from build123d import *

# Parameters (mm, degrees)
F4_D     = 2.5
F4_DEPTH = 8
F4_START = 17.6049004
F4_TIP   = 0.7510757738


with BuildPart() as f1:
    # F0 (on Front) → F1 (revolve)
    with BuildSketch(Plane.XZ):
        Polygon((-7.5, 3), (13.5, 3), (13.5, 4), (7.5, 4), (7.5, 10), (5.75, 10), (5.75, 7.5), (-5.75, 7.5), (-5.75, 10), (-7.5, 10), align=None)
    revolve(axis=Axis((1.1428869498, 0, 0), (1, 0, 0)))

    # F4
    # its depths count from where the whole tool has entered the part; down to there all is cleared
    with Locations(Plane.XY.offset(25)):
        with Locations((0, 0)):
            Hole(F4_D / 2, depth=F4_START)
    with Locations(Plane.XY.offset(25).offset(-F4_START)):
        with Locations((0, 0)):
            Hole(F4_D / 2, depth=F4_DEPTH)
            with Locations((0, 0, -(F4_DEPTH + F4_TIP / 2))):  # 118° drill point
                Cone(0, F4_D / 2, F4_TIP, mode=Mode.SUBTRACT)


solid = f1.part
Work out the finished part from the listing and answer in its coordinate system (mm). A direction names the side the tool comes from. Give positions to 0.01 mm unless a question says otherwise; leave off trailing zeros. Order: outer loops, then holes, each group sorted by start corner. A loop starts at its lowest first (then second) coordinate and runs counter-clockwise, first axis right, second up. Notation, with made-up numbers: M -38.5,78.5 L -4.5,78.5 A30 cw -4.5,112.5 Z; hole C 56.25,27 d8. An arc over 180 degrees is marked long. Return JSON: item names as keys, results as strings.
Q1. The mould has two halves that part along Z. Classify faces 6 (the face through (6.61, 9.76, -2.17)), 7 (the face through (7.5, -0.1, -4.3)), 8 (the face through (3.1, 1.8, -2.4)): pulls with the +Z half, pulls with the -Z half, needs draft (parallel to the pull), parting line crosses it, or undercut.
Answer below:
{"face 6": "parting line crosses it", "face 7": "needs draft", "face 8": "undercut"}
Q2. Which of the six approach directions +Z, -Z, +X, -X, +Y, -Y give full straight-line access (tool end or side, diameter ignored) to faces 1 (the face through (-6.64, 9.76, -2.17)), 2 (the face through (10.458, 3.905, -0.867)), 3 (the face through (-0.59, 1.1, 5.08)), 4 (the face through (-5.75, -7, -4)), 5 (the face through (-7.5, -2.4, 2.1))?
Answer below:
{"face 1": "+X, -X", "face 2": "+X", "face 3": "+Z", "face 4": "none", "face 5": "+Z, -Z, -X, +Y, -Y"}
Q3. Each of these flat-tipped pins is pushed along its axis until it touches: pin 1 (6 mm diameter, centred on x = 1, z = -3.5, fed in from -Y); pin 2 (4 mm diameter, centred on y = 6.5, z = 7, fed in from +X); pin 3 (8 mm diameter, centred on x = 1.5, y = 8, fed in from +Z). Where does it stop, or does it pass through?
Answer below:
{"pin 1": "stops at y = -7.48", "pin 2": "stops at x = 7.5", "pin 3": "stops at z = 6.34"}
Q4. Find the intervals of material crossed by line 1 along Y through (x, z) = (8.75, 0); line 2 along X through (y, z) = (7.25, 2.75); line 3 along Y through (x, z) = (3, 0), in increasing order. Write a range as [from, to].
Answer below:
{"line 1": "y = [-4, -3], [3, 4]", "line 2": "x = [-7.5, -5.75], [5.75, 7.5]", "line 3": "y = [-7.5, -3], [3, 7.5]"}
Q5. Find section C-C, the plane y = -8.25. Write down the section's boundary in (x, z), and give its area (3 significant figures).
Answer below:
{"outline": "M -7.5,-5.65 L -5.75,-5.65 L -5.75,5.65 L -7.5,5.65 Z; M 5.75,-5.65 L 7.5,-5.65 L 7.5,5.65 L 5.75,5.65 Z", "area": "39.6 mm^2"}
Q6. Find section A-A, the plane z = 0. Write down the section's boundary in (x, y).
Answer below:
{"outline": "M -7.5,-10 L -5.75,-10 L -5.75,-7.5 L 5.75,-7.5 L 5.75,-10 L 7.5,-10 L 7.5,-4 L 13.5,-4 L 13.5,-3 L -7.5,-3 Z; M -7.5,3 L 13.5,3 L 13.5,4 L 7.5,4 L 7.5,10 L 5.75,10 L 5.75,7.5 L -5.75,7.5 L -5.75,10 L -7.5,10 Z"}
Q7. Find section D-D, the plane x = -2.5. Write down the section's boundary in (y, z), and give its area (3 significant figures).
Answer below:
{"outline": "C 0,0 d15; hole C 0,0 d6", "area": "148 mm^2"}
Q8. Find section B-B, the plane y = 0. Write down the section's boundary in (x, z), and give its area (3 significant figures).
Answer below:
{"outline": "M -7.5,-10 L -5.75,-10 L -5.75,-7.5 L 5.75,-7.5 L 5.75,-10 L 7.5,-10 L 7.5,-4 L 13.5,-4 L 13.5,-3 L -7.5,-3 Z; M -7.5,3 L -1.25,3 L -1.25,7.5 L -5.75,7.5 L -5.75,10 L -7.5,10 Z; M 1.25,3 L 13.5,3 L 13.5,4 L 7.5,4 L 7.5,10 L 5.75,10 L 5.75,7.5 L 1.25,7.5 Z", "area": "153 mm^2"}
